Autodesk Inventor part; units mm, degrees
ref_plane "YZ Plane" through (0, 0, 0) normal (1, 0, 0) x (0, 1, 0)
ref_plane "XZ Plane" through (0, 0, 0) normal (0, 1, 0) x (-1, 0, 0)
ref_plane "XY Plane" through (0, 0, 0) normal (0, 0, 1) x (1, 0, 0)
sketch "Sketch1" plane through (0, 0, 0) normal (0, 0, 1) x (1, 0, 0)
  arc A0 (-37.287, 7.8288) -> (37.287, 7.8288) centre (0, 0) ccw
  arc A1 (18.6435, 96.6244) -> (-18.6435, 96.6244) centre (0, 92.71) ccw
  line L0 (-18.6435, 96.6244) -> (-37.287, 7.8288)
  line L1 (18.6435, 96.6244) -> (37.287, 7.8288)
  dimension "d0" = 76.2
  dimension "d1" = 38.1
  dimension "d2" = 149.86
extrude "Extrusion1" add sketch "Sketch1" along normal blind 20.32
shell "Shell1" thickness 2.54 removed faces 1 at (-6.2145, 37.4273, 20.32)
sketch "Sketch2" plane through (0, 0, 0) normal (0, 0, -1) x (-1, 0, 0)
  circle A0 centre (0, 0) radius 5.969
  arc A1 (-37.287, 7.8288) -> (37.287, 7.8288) centre (0, 0) ccw
  circle A2 centre (0, 0) radius 10.795
  dimension "d6" = 11.938
  dimension "d7" = 21.59
extrude "Extrusion2" add sketch "Sketch2" along normal blind 7.62
hole "Hole1" at (0, 0, 0) direction (0, 0, 1) diameter 11.938 end through all
properties part number "ChainGuard"
Build history of the part. All positions in model axes, mm. A direction names the side the tool comes from. Round coordinates to 2 decimals unless told otherwise and drop trailing zeros. Loops run counter-clockwise (first coordinate to the right, second up) from the corner with the lowest first, then second, coordinate; pieces in that order, holes last. Notation, with made-up numbers: (2, -38.5) -> (35, -38.5) arc R13 ccw to (35, -25.5) -> close; hole circle Ø9 at (17.25, 74). An arc over 180 degrees is marked (long way). Answer in a Markdown table with one row per item.
Item 1: Saw through at A-A (x = 0). Write the cut outline in (y, z) (3 decimals), and give its area (3 significant figures).
Answers below:
| item | result |
|---|---|
| outline | (-38.1, 0) -> (-10.795, 0) -> (-10.795, -7.62) -> (-5.969, -7.62) -> (-5.969, 2.54) -> (-35.56, 2.54) -> (-35.56, 20.32) -> (-38.1, 20.32) -> close; (5.969, -7.62) -> (10.795, -7.62) -> (10.795, 0) -> (111.76, 0) -> (111.76, 20.32) -> (109.22, 20.32) -> (109.22, 2.54) -> (5.969, 2.54) -> close |
| area | 514 mm² |
Item 2: Which spindle directions (+Z, -Z, +X, -X, +Y, -Y) get a long thin tool onto all of the face, cutting with end or side? Do faces 1 (the flat face through (28, 43, 20.32)), 2 (the flat face through (25.35, 52.33, 11.31)). Say none if no direction does.
Answers below:
| item | result |
|---|---|
| face 1 | +Z, +X, -X, +Y, -Y |
| face 2 | +Z |
Item 3: Drill centre lines: L1, parallel to Y at x = 0, z = 0.75; L2, parallel to Y at x = 0, z = 8; L3, parallel to X at y = 0, z = 7.25. Where is each one in solid material? Low to high. Write a range as [from, to].
Answers below:
| item | result |
|---|---|
| L1 | y = [-38.1, -5.97], [5.97, 111.76] |
| L2 | y = [-38.1, -35.56], [109.22, 111.76] |
| L3 | x = [-38.1, -35.56], [35.56, 38.1] |
Item 4: Saw through at B-B (y = 0). Write the cut outline in (x, z) (3 decimals).
Answers below:
| item | result |
|---|---|
| outline | (-38.1, 0) -> (-10.795, 0) -> (-10.795, -7.62) -> (-5.969, -7.62) -> (-5.969, 2.54) -> (-35.56, 2.54) -> (-35.56, 20.32) -> (-38.1, 20.32) -> close; (5.969, -7.62) -> (10.795, -7.62) -> (10.795, 0) -> (38.1, 0) -> (38.1, 20.32) -> (35.56, 20.32) -> (35.56, 2.54) -> (5.969, 2.54) -> close |
Item 5: Pin check, flat tips, straight feed: pin 1 (5 mm diameter, centred on y = 33.5, z = 6, fed in from +X); pin 2 (1 mm diameter, centred on x = -18, y = 66, fed in from -Z); pin 3 (6 mm diameter, centred on x = -10.5, z = 12.5, fed in from +Y). Stop position of each tip, or through.
Answers below:
| item | result |
|---|---|
| pin 1 | stops at x = 32.42 |
| pin 2 | stops at z = 0 |
| pin 3 | stops at y = 110.22 |
Item 6: Saw through at D-D (x = 31.5). Write the cut outline in (y, z), and give its area (3 significant figures).
Answers below:
| item | result |
|---|---|
| outline | (-21.43, 0) -> (35.39, 0) -> (35.39, 20.32) -> (23.03, 20.32) -> (23.03, 2.54) -> (-16.5, 2.54) -> (-16.5, 20.32) -> (-21.43, 20.32) -> close |
| area | 452 mm² |
Item 7: Saw through at C-C (z = 5). Write the cut outline in (x, y), and give its area (3 significant figures).
Answers below:
| item | result |
|---|---|
| outline | (-37.29, 7.83) arc R38.1 ccw (long way) to (37.29, 7.83) -> (18.64, 96.62) arc R19.05 ccw to (-18.64, 96.62) -> close; hole (-34.8, 7.31) arc R35.56 ccw (long way) to (34.8, 7.31) -> (16.16, 96.1) arc R16.51 ccw to (-16.16, 96.1) -> close |
| area | 917 mm² |
Item 8: Mould opens along Y. For faces 3 (the cylindrical face through (7.956, -7.296, -3.757)), 4 (the flat face through (-5, -5, -7.62)), 5 (the flat face through (0, 22, 2.54)) say: +Y half, -Y half, draft (parallel to the pull), parting line (faces both ways), or undercut.
Answers below:
| item | result |
|---|---|
| face 3 | parting line |
| face 4 | draft |
| face 5 | undercut |
